```python
from build123d import *

# Parameters (mm, degrees)
SKETCH1_W           = 165.1
SKETCH1_H           = 139.7
BOSS_EXTRUDE1_DEPTH = 6.35
SKETCH2_W           = 50.8
SKETCH2_H           = 50.8
BOSS_EXTRUDE2_DEPTH = 127
CUT_EXTRUDE1_DEPTH  = 184.491927615
FILLET1_R           = 10
MIRROR6_START       = -25.4
MIRROR6_DEPTH       = 50.8
CUT_EXTRUDE2_DEPTH  = 127


with BuildPart() as part:
    # Sketch1 → Boss-Extrude1 (new body)
    with BuildSketch(Plane(origin=(0, 0, 0), x_dir=(1, 0, 0), z_dir=(0, 1, 0))):
        Rectangle(SKETCH1_W, SKETCH1_H)
    extrude(amount=BOSS_EXTRUDE1_DEPTH)

    # Sketch2 → Boss-Extrude2 (add)
    with BuildSketch(Plane(origin=(0, 6.35, 0), x_dir=(1, 0, 0), z_dir=(0, 1, 0))):
        with Locations((50.8, 0)):
            Rectangle(SKETCH2_W, SKETCH2_H)
    extrude(amount=BOSS_EXTRUDE2_DEPTH)

    # Sketch4 → Cut-Extrude1 (cut, through all)
    with BuildSketch(Plane.XY.offset(25.4)):
        Polygon((31.75, 133.35), (31.75, 19.05), (76.2, 12.7), (95.954687833, 12.7), (95.954687833, 161.138699607), (31.75, 161.138699607), align=None)
    extrude(amount=-CUT_EXTRUDE1_DEPTH, mode=Mode.SUBTRACT)

    # Fillet1
    # the kernel refuses this fillet: 10 mm, written as the material it adds along each edge
    with BuildSketch(Plane(origin=(31.75, 19.05, 25.4), x_dir=(0.9899494936611666, -0.14142135623730998, 0), z_dir=(0, 0, -1))) as fillet1_piece_1:
        with BuildLine():
            CenterArc((FILLET1_R * 0.867295401695, -FILLET1_R), FILLET1_R, 90, 81.869897646)
            Line((-FILLET1_R * 0.122654091966, -FILLET1_R * 0.858578643763), (0, 0))
            Line((0, 0), (FILLET1_R * 0.867295401695, 0))
        make_face()
    extrude(amount=50.8)
    # the kernel refuses this fillet: 10 mm, written as the material it takes off along each edge
    with BuildSketch(Plane(origin=(76.2, 12.7, 46.366939289), x_dir=(0, -1, 0), z_dir=(0, 0, -1))) as fillet1_2_piece_1:
        with BuildLine():
            CenterArc((8.71342574, 9.716697935), FILLET1_R, 188.130102354, 68.199121512)
            Line((-1.186069196, 8.302484373), (0, 0))
            Line((0, 0), (6.35, 0))
        make_face()
    extrude(amount=92.733878578, mode=Mode.SUBTRACT)
    with BuildSketch(Plane(origin=(31.75, 133.35, 48.675187969), x_dir=(-1, 0, 0), z_dir=(0, 0, -1))) as fillet1_2_piece_2:
        with BuildLine():
            CenterArc((10, -9.310075188), FILLET1_R, 111.407582704, 68.592417296)
            Line((0, -9.310075188), (0, 0))
            Line((0, 0), (6.35, 0))
        make_face()
    extrude(amount=97.350375938, mode=Mode.SUBTRACT)

    # Mirror6: read off the stored shape, not the designer's step
    # Mirror6 outline → Mirror6 (add)
    with BuildSketch(Plane.XY.offset(MIRROR6_START)):
        with BuildLine():
            Line((-76.2, 6.35), (-25.4, 6.35))
            Line((-25.4, 6.35), (-25.4, 133.35))
            ThreePointArc((-25.4, 133.35), (-30.011355821, 129.674638647), (-31.75, 124.039924812))
            Line((-31.75, 124.039924812), (-31.75, 27.722954017))
            ThreePointArc((-31.75, 27.722954017), (-34.19546045, 21.170936603), (-40.335786438, 17.82345908))
            Line((-40.335786438, 17.82345908), (-67.897515627, 13.886069196))
            ThreePointArc((-67.897515627, 13.886069196), (-73.204342343, 11.391141605), (-76.2, 6.35))
        make_face()
    extrude(amount=MIRROR6_DEPTH)

    # Sketch6 → Cut-Extrude2 (cut)
    with BuildSketch(Plane(origin=(0, 6.35, 0), x_dir=(-1, 0, 0), z_dir=(0, 1, 0))):
        with BuildLine():
            Line((-41.275, 48.8188), (-66.675, 48.8188))
            ThreePointArc((-66.675, 48.8188), (-71.8312, 53.975), (-66.675, 59.1312))
            Line((-66.675, 59.1312), (-41.275, 59.1312))
            ThreePointArc((-41.275, 59.1312), (-36.1188, 53.975), (-41.275, 48.8188))
        make_face()
        with BuildLine():
            Line((-41.275, -59.1312), (-66.675, -59.1312))
            ThreePointArc((-66.675, -59.1312), (-71.8312, -53.975), (-66.675, -48.8188))
            Line((-66.675, -48.8188), (-41.275, -48.8188))
            ThreePointArc((-41.275, -48.8188), (-36.1188, -53.975), (-41.275, -59.1312))
        make_face()
        with BuildLine():
            Line((41.275, 59.1312), (66.675, 59.1312))
            ThreePointArc((66.675, 59.1312), (71.8312, 53.975), (66.675, 48.8188))
            Line((66.675, 48.8188), (41.275, 48.8188))
            ThreePointArc((41.275, 48.8188), (36.1188, 53.975), (41.275, 59.1312))
        make_face()
        with BuildLine():
            Line((41.275, -48.8188), (66.675, -48.8188))
            ThreePointArc((66.675, -48.8188), (71.8312, -53.975), (66.675, -59.1312))
            Line((66.675, -59.1312), (41.275, -59.1312))
            ThreePointArc((41.275, -59.1312), (36.1188, -53.975), (41.275, -48.8188))
        make_face()
    extrude(amount=-CUT_EXTRUDE2_DEPTH, mode=Mode.SUBTRACT)


solid = part.part
```
CAD build for the part. Positions are in the model's coordinates, mm. A direction names the side the tool comes from. Round coordinates to 2 decimals unless told otherwise and drop trailing zeros. Write each loop counter-clockwise with the first axis right and the second up, starting at its lowest first coordinate (ties: lowest second). Pieces come first, ordered by that corner, then holes. Notation, with made-up numbers: (39.25, 28.25) - (68.25, 28.25) arc R26 cw to (68.25, 59.25) - close; hole circle Ø6 at (13.5, -13.5). An arc over 180 degrees is marked (long way). Return JSON: item names as keys, results as strings. Group by question number.
Item 1: Mould opens along Z. For faces 5 (the face through (-1, 6.35, -1)), 6 (the face through (-1, 3, 69.85)), 7 (the face through (54, 3, -48.819)), 8 (the face through (54, 3, -59.131)) say: +Z half, -Z half, draft (parallel to the pull), parting line (faces both ways), or undercut.
Item 2: Probe probe 1 along X at (y, z) = (71, 4); probe 2 along Y at (x, z) = (32.5, -27.5); probe 3 along X at (y, z) = (126, 5.5). List the from-to ranges inside material, lowest first.
Item 3: Band-saw the part on D-D on z = -52. List the corners of the cut face in (x, y).
Item 4: Flat gauge pins, fed straight in: pin 1 Ø1 at (x, y) = (27.5, 104.5) entering from +Z; pin 2 Ø3 at (x, z) = (40.5, 15.5) entering from +Y; pin 3 Ø5 at (y, z) = (110.5, 7.5) entering from -X; pin 4 Ø8 at (x, z) = (-19, 7) entering from -Y. Where does each tip first touch, or does it go through?
Item 5: Band-saw the part on B-B on z = -11. List the corners of the cut face in (x, y), plus the area to 3 significant figures.
Item 6: Band-saw the part on A-A on y = 31. List the corners of the cut face in (x, z).
Item 7: Band-saw the part on C-C on x = -59.5. List the corners of the cut face in (y, z).
Item 8: 3-axis set-ups, long thin cutter, end or side, ignore diameter. For faces 1 (the face through (-30, 42, -25.4)), 2 (the face through (-25.4, 69, 0)), 3 (the face through (-54, 3, -59.131)), 4 (the face through (31.75, 77, 0)): which of +Z, -Z, +X, -X, +Y, -Y reach the whole face in a straight line?
Resolved:
{
 "1": {"face 5": "draft", "face 6": "+Z half", "face 7": "undercut", "face 8": "undercut"},
 "2": {"probe 1": "x = -31.75 to -25.4, 25.4 to 31.75", "probe 2": "y = 0 to 6.35", "probe 3": "x = -31.56 to -25.4, 25.4 to 31.56"},
 "3": {"outline": "(-82.55, 0) - (-71.44, 0) - (-71.44, 6.35) - (-82.55, 6.35) - close; (-36.51, 0) - (36.51, 0) - (36.51, 6.35) - (-36.51, 6.35) - close; (71.44, 0) - (82.55, 0) - (82.55, 6.35) - (71.44, 6.35) - close"},
 "4": {"pin 1": "stops at z = 25.4", "pin 2": "stops at y = 18.11", "pin 3": "stops at x = -31.75", "pin 4": "stops at y = 0"},
 "5": {"outline": "(-82.55, 0) - (82.55, 0) - (82.55, 6.35) - (76.2, 6.35) arc R10 ccw to (67.9, 13.89) - (40.34, 17.82) arc R10 cw to (31.75, 27.72) - (31.75, 124.04) arc R10 ccw to (25.4, 133.35) - (25.4, 6.35) - (-25.4, 6.35) - (-25.4, 133.35) arc R10 ccw to (-31.75, 124.04) - (-31.75, 27.72) arc R10 cw to (-40.34, 17.82) - (-67.9, 13.89) arc R10 ccw to (-76.2, 6.35) - (-82.55, 6.35) - close", "area": "3,480 mm²"},
 "6": {"outline": "(-31.75, -25.4) - (-25.4, -25.4) - (-25.4, 25.4) - (-31.75, 25.4) - close; (25.4, -25.4) - (31.75, -25.4) - (31.75, 25.4) - (25.4, 25.4) - close"},
 "7": {"outline": "(0, -69.85) - (6.35, -69.85) - (6.35, -59.13) - (0, -59.13) - close; (0, -48.82) - (6.35, -48.82) - (6.35, -25.4) - (15.09, -25.4) - (15.09, 25.4) - (6.35, 25.4) - (6.35, 48.82) - (0, 48.82) - close; (0, 59.13) - (6.35, 59.13) - (6.35, 69.85) - (0, 69.85) - close"},
 "8": {"face 1": "-Z, +X, -X, +Y", "face 2": "+Z, -Z, +Y", "face 3": "+Y, -Y", "face 4": "+Z, -Z, +X, +Y"}
}
